```python
from build123d import *

# Parameters (mm, degrees)
ESQUISSE1_W             = 200
ESQUISSE1_H             = 300
BOSS_EXTRU_1_DEPTH      = 80
COQUE1_T                = -6
ESQUISSE3_W             = 194.2
ESQUISSE3_H             = 294.2
ENL_V_MAT_EXTRU_2_DEPTH = 6.1
ESQUISSE4_R             = 9
BOSS_EXTRU_2_DEPTH      = 67.9
ESQUISSE5_R             = 2.5
ENL_V_MAT_EXTRU_3_DEPTH = 30
ESQUISSE4_4_R           = 9
BOSS_EXTRU_3_DEPTH      = 15
ESQUISSE6_R             = 2.5
ENL_V_MAT_EXTRU_6_DEPTH = 10
ESQUISSE8_R             = 9
BOSS_EXTRU_5_DEPTH      = 68
ESQUISSE9_R             = 2.5
ENL_V_MAT_EXTRU_8_DEPTH = 30


with BuildPart() as part:
    # Esquisse1 → Boss.-Extru.1 (new body)
    with BuildSketch(Plane.XY):
        with Locations((43.373964051, -118.711656442)):
            Rectangle(ESQUISSE1_W, ESQUISSE1_H)
    extrude(amount=BOSS_EXTRU_1_DEPTH)

    # Coque1
    coque1_openings = [part.faces().sort_by_distance(p)[0] for p in [
        (43.373964051, -118.711656442, 0),
    ]]
    offset(amount=COQUE1_T, openings=coque1_openings, kind=Kind.INTERSECTION)

    # Esquisse3 → Enl_v. mat.-Extru.2 (cut)
    with BuildSketch(Plane(origin=(0, 0, 0), x_dir=(-1, 0, 0), z_dir=(0, 0, -1))):
        with Locations((-43.373964051, -118.711656442)):
            Rectangle(ESQUISSE3_W, ESQUISSE3_H)
    extrude(amount=-ENL_V_MAT_EXTRU_2_DEPTH, mode=Mode.SUBTRACT)

    # Esquisse4 → Boss.-Extru.2 (add)
    with BuildSketch(Plane(origin=(0, 0, 74), x_dir=(-1, 0, 0), z_dir=(0, 0, -1))):
        with Locations((-117.373964051, 5.288343558)):
            Circle(ESQUISSE4_R)
    extrude(amount=BOSS_EXTRU_2_DEPTH)

    # Esquisse5 → Enl_v. mat.-Extru.3 (cut)
    with BuildSketch(Plane(origin=(0, 0, 6.1), x_dir=(-1, 0, 0), z_dir=(0, 0, -1))):
        with Locations((-117.373964051, 5.288343558)):
            Circle(ESQUISSE5_R)
    extrude(amount=-ENL_V_MAT_EXTRU_3_DEPTH, mode=Mode.SUBTRACT)

    # Esquisse4_4 → Boss.-Extru.3 (add)
    with BuildSketch(Plane(origin=(0, 0, 74), x_dir=(-1, 0, 0), z_dir=(0, 0, -1))):
        with BuildLine():
            Line((-99.873964051, -44.711656442), (-99.873964051, -53.711656442))
            Line((-99.873964051, -53.711656442), (-108.873964051, -53.711656442))
            ThreePointArc((-108.873964051, -53.711656442), (-99.873964051, -62.711656442), (-90.873964051, -53.711656442))
            ThreePointArc((-90.873964051, -53.711656442), (-93.510003021, -47.347695411), (-99.873964051, -44.711656442))
        make_face()
        with BuildLine():
            Line((-108.873964051, -53.711656442), (-99.873964051, -53.711656442))
            Line((-99.873964051, -53.711656442), (-99.873964051, -44.711656442))
            ThreePointArc((-99.873964051, -44.711656442), (-106.237925082, -47.347695411), (-108.873964051, -53.711656442))
        make_face()
        with BuildLine():
            Line((-99.873964051, -44.711656442), (-99.873964051, -53.711656442))
            Line((-99.873964051, -53.711656442), (-108.873964051, -53.711656442))
            ThreePointArc((-108.873964051, -53.711656442), (-99.873964051, -62.711656442), (-90.873964051, -53.711656442))
            ThreePointArc((-90.873964051, -53.711656442), (-93.510003021, -47.347695411), (-99.873964051, -44.711656442))
        make_face()
        with BuildLine():
            Line((-108.873964051, -53.711656442), (-99.873964051, -53.711656442))
            Line((-99.873964051, -53.711656442), (-99.873964051, -44.711656442))
            ThreePointArc((-99.873964051, -44.711656442), (-106.237925082, -47.347695411), (-108.873964051, -53.711656442))
        make_face()
        with BuildLine():
            Line((13.126035949, -192.711656442), (13.126035949, -183.711656442))
            Line((13.126035949, -183.711656442), (22.126035949, -183.711656442))
            ThreePointArc((22.126035949, -183.711656442), (6.762074918, -177.347695411), (13.126035949, -192.711656442))
        make_face()
        with BuildLine():
            Line((22.126035949, -183.711656442), (13.126035949, -183.711656442))
            Line((13.126035949, -183.711656442), (13.126035949, -192.711656442))
            ThreePointArc((13.126035949, -192.711656442), (19.489996979, -190.075617472), (22.126035949, -183.711656442))
        make_face()
        with BuildLine():
            Line((13.126035949, -192.711656442), (13.126035949, -183.711656442))
            Line((13.126035949, -183.711656442), (22.126035949, -183.711656442))
            ThreePointArc((22.126035949, -183.711656442), (6.762074918, -177.347695411), (13.126035949, -192.711656442))
        make_face()
        with BuildLine():
            Line((22.126035949, -183.711656442), (13.126035949, -183.711656442))
            Line((13.126035949, -183.711656442), (13.126035949, -192.711656442))
            ThreePointArc((13.126035949, -192.711656442), (19.489996979, -190.075617472), (22.126035949, -183.711656442))
        make_face()
        with Locations((13.126035949, -53.711656442)):
            Circle(ESQUISSE4_4_R)
        with Locations((-99.873964051, -183.711656442)):
            Circle(ESQUISSE4_4_R)
    extrude(amount=BOSS_EXTRU_3_DEPTH)

    # Esquisse6 → Enl_v. mat.-Extru.6 (cut)
    with BuildSketch(Plane(origin=(0, 0, 59), x_dir=(-1, 0, 0), z_dir=(0, 0, -1))):
        with Locations((-99.873964051, -53.711656442)):
            Circle(ESQUISSE6_R)
        with Locations((13.126035949, -53.711656442)):
            Circle(ESQUISSE6_R)
        with Locations((-99.873964051, -183.711656442)):
            Circle(ESQUISSE6_R)
        with Locations((13.126035949, -183.711656442)):
            Circle(ESQUISSE6_R)
    extrude(amount=-ENL_V_MAT_EXTRU_6_DEPTH, mode=Mode.SUBTRACT)

    # Esquisse8 → Boss.-Extru.5 (add)
    with BuildSketch(Plane(origin=(0, 0, 74), x_dir=(-1, 0, 0), z_dir=(0, 0, -1))):
        with BuildLine():
            Line((30.626035949, 14.288343558), (30.626035949, 5.288343558))
            Line((30.626035949, 5.288343558), (39.626035949, 5.288343558))
            ThreePointArc((39.626035949, 5.288343558), (36.989996979, 11.652304589), (30.626035949, 14.288343558))
        make_face()
        with BuildLine():
            Line((39.626035949, 5.288343558), (30.626035949, 5.288343558))
            Line((30.626035949, 5.288343558), (30.626035949, 14.288343558))
            ThreePointArc((30.626035949, 14.288343558), (24.262074918, -1.075617472), (39.626035949, 5.288343558))
        make_face()
        with BuildLine():
            Line((30.626035949, 14.288343558), (30.626035949, 5.288343558))
            Line((30.626035949, 5.288343558), (39.626035949, 5.288343558))
            ThreePointArc((39.626035949, 5.288343558), (36.989996979, 11.652304589), (30.626035949, 14.288343558))
        make_face()
        with BuildLine():
            Line((39.626035949, 5.288343558), (30.626035949, 5.288343558))
            Line((30.626035949, 5.288343558), (30.626035949, 14.288343558))
            ThreePointArc((30.626035949, 14.288343558), (24.262074918, -1.075617472), (39.626035949, 5.288343558))
        make_face()
        with BuildLine():
            Line((30.626035949, -251.711656442), (30.626035949, -242.711656442))
            Line((30.626035949, -242.711656442), (39.626035949, -242.711656442))
            ThreePointArc((39.626035949, -242.711656442), (24.262074918, -236.347695411), (30.626035949, -251.711656442))
        make_face()
        with BuildLine():
            Line((39.626035949, -242.711656442), (30.626035949, -242.711656442))
            Line((30.626035949, -242.711656442), (30.626035949, -251.711656442))
            ThreePointArc((30.626035949, -251.711656442), (36.989996979, -249.075617472), (39.626035949, -242.711656442))
        make_face()
        with BuildLine():
            Line((30.626035949, -251.711656442), (30.626035949, -242.711656442))
            Line((30.626035949, -242.711656442), (39.626035949, -242.711656442))
            ThreePointArc((39.626035949, -242.711656442), (24.262074918, -236.347695411), (30.626035949, -251.711656442))
        make_face()
        with BuildLine():
            Line((39.626035949, -242.711656442), (30.626035949, -242.711656442))
            Line((30.626035949, -242.711656442), (30.626035949, -251.711656442))
            ThreePointArc((30.626035949, -251.711656442), (36.989996979, -249.075617472), (39.626035949, -242.711656442))
        make_face()
        with Locations((-117.373964051, -242.711656442)):
            Circle(ESQUISSE8_R)
    extrude(amount=BOSS_EXTRU_5_DEPTH)

    # Esquisse9 → Enl_v. mat.-Extru.8 (cut)
    with BuildSketch(Plane(origin=(0, 0, 6), x_dir=(-1, 0, 0), z_dir=(0, 0, -1))):
        with Locations((30.626035949, 5.288343558)):
            Circle(ESQUISSE9_R)
        with Locations((30.626035949, -242.711656442)):
            Circle(ESQUISSE9_R)
        with Locations((-117.373964051, -242.711656442)):
            Circle(ESQUISSE9_R)
    extrude(amount=-ENL_V_MAT_EXTRU_8_DEPTH, mode=Mode.SUBTRACT)


with BuildPart() as part_1:
    # Corps-D_placer_Copier1: moved
    add(part.part.moved(Location((0, 114, 0))))


with BuildPart() as part_2:
    # Corps-D_placer_Copier2: moved
    add(part_1.part.moved(Location((0, 20, 0))))


solid = part_2.part
```
Geometry check sheet. Reference: the model listing, model coordinates, mm. A direction names the side the tool comes from. Give positions to 0.01 mm unless a question says otherwise; leave off trailing zeros. Loops run counter-clockwise (first coordinate to the right, second up) from the corner with the lowest first, then second, coordinate; pieces in that order, holes last. Notation, with made-up numbers: M 84.25,-34.75 L 91.25,-34.75 A34 cw 91.25,-1.75 Z; hole C 66,36.25 d3. An arc over 180 degrees is marked long. Write item = value, one per line. Start each with the question number.
1. Section check B-B, the plane z = 15. Give the number of separate pieces and of enclosed holes in the cut face, plus the area to 3 significant figures.
2. Go/stop test with flat-tipped pins: P1, Ø1.5, axis at x = -14, y = -49, coming from the -Z side; P2, Ø5.5, axis at x = 99, y = 80.5, coming from the -Z side; P3, Ø4, axis at x = 118.5, y = 139.5, coming from the -Z side. Record where each tip stops, or that it passes through.
3. Tool access check on faces 5 (the face through (45, 162.388, 3)), 6 (the face through (143.374, 13, 39)). Record the directions out of +Z, -Z, +X, -X, +Y, -Y that give a thin tool (end or side, any length) a straight path to the whole face; none if there is none.
4. Draft check along Y on faces 1 (the face through (42, 165.288, 39)), 2 (the face through (-50.626, 13, 40)), 3 (the face through (-56.626, 13, 39)), 4 (the face through (126.365, 139.684, 40.525)). Enter one of: +Y half, -Y half, draft (parallel to the pull), parting line (faces both ways), or undercut.
5. Section check C-C, the plane y = 103.5. Enter the section's corners in (x, z), plus the area to 3 significant figures.
6. Thickness scan on probe 1 along X at (y, z) = (79, 22); probe 2 along Y at (x, z) = (-30, 69); probe 3 along Y at (x, z) = (46.5, 25). Record the ranges inside material, lowest first.
7. Section check D-D, the plane x = 85. Enter the section's corners in (y, z).
8. Section check A-A, the plane z = 47. Enter the section's corners in (x, y), plus the area to 3 significant figures.
Values follow:
q1.separate_pieces = 5
q1.enclosed_holes = 5
q1.area = 6,800 mm^2
q2.P1 = 69
q2.P2 = 59
q2.P3 = 6.1
q3.face_5 = -Z
q3.face_6 = +Z, -Z, +X, +Y, -Y
q4.face_1 = +Y half
q4.face_2 = undercut
q4.face_3 = draft
q4.face_4 = undercut
q5.outline = M -56.63,0 L -53.73,0 L -53.73,6.1 L -50.63,6.1 L -50.63,74 L 137.37,74 L 137.37,6.1 L 140.47,6.1 L 140.47,0 L 143.37,0 L 143.37,80 L -56.63,80 Z
q5.area = 2,050 mm^2
q6.probe_1 = -56.63 to -50.63, 137.37 to 143.37
q6.probe_2 = -134.71 to -128.71, -117.69 to -99.73, 130.31 to 148.27, 159.29 to 165.29
q6.probe_3 = -134.71 to -128.71, 159.29 to 165.29
q7.outline = M -134.71,0 L -131.81,0 L -131.81,6.1 L -128.71,6.1 L -128.71,74 L 159.29,74 L 159.29,6.1 L 162.39,6.1 L 162.39,0 L 165.29,0 L 165.29,80 L -134.71,80 Z
q8.outline = M -56.63,-134.71 L 143.37,-134.71 L 143.37,165.29 L -56.63,165.29 Z; C -30.63,-108.71 d18; C -30.63,139.29 d18; C 117.37,-108.71 d18; C 117.37,139.29 d18; hole M -50.63,-128.71 L 137.37,-128.71 L 137.37,159.29 L -50.63,159.29 Z
q8.area = 6,870 mm^2
